Input: part model. Units: mm. Frame: model coordinates. Give positions to 0.01 mm unless a question says otherwise; leave off trailing zeros. Loops run counter-clockwise (first coordinate to the right, second up) from the corner with the lowest first, then second, coordinate; pieces in that order, holes last.
Autodesk Inventor part; units mm, degrees
ref_plane "YZ Plane" through (0, 0, 0) normal (1, 0, 0) x (0, 1, 0)
ref_plane "XZ Plane" through (0, 0, 0) normal (0, 1, 0) x (-1, 0, 0)
ref_plane "XY Plane" through (0, 0, 0) normal (0, 0, 1) x (1, 0, 0)
sketch "スケッチ1" plane through (0, 0, 0) normal (0, 0, 1) x (1, 0, 0)
  line L0 (-18.5, 36) -> (18.5, 36)
  line L1 (18.5, 36) -> (18.5, 0)
  line L2 (18.5, 0) -> (-18.5, 0)
  line L3 (-18.5, 0) -> (-18.5, 36)
  circle A0 centre (0, 4) radius 1.6
  circle A1 centre (14, 32) radius 1.6
  circle A2 centre (-14, 32) radius 1.6
  line L4 (0, 42.25) -> (0, -4.7356) construction
  point P0 (0, 0)
  point P1 (0, 0)
  dimension "d0" = 37
  dimension "d1" = 36
  dimension "d2" = 3.2
  dimension "d3" = 4
  dimension "d4" = 4
  dimension "d5" = 4.5
extrude "押し出し1" add sketch "スケッチ1" along normal blind 1.6
properties part number "PCB-EncoderMain"
(1) Ray query, probe 1 along Y at (x, z) = (14, 0.95); probe 2 along Y at (x, z) = (0, 0.9); probe 3 along X at (y, z) = (3, 0.55). Return the intervals inside material, ascending.
Values follow:
probe 1: y = 0 to 30.4, 33.6 to 36
probe 2: y = 0 to 2.4, 5.6 to 36
probe 3: x = -18.5 to -1.25, 1.25 to 18.5
(2) Cut plane B-B (x = 0). Return the cut outline in (y, z).
Values follow:
outline: (0, 0) - (2.4, 0) - (2.4, 1.6) - (0, 1.6) - close; (5.6, 0) - (36, 0) - (36, 1.6) - (5.6, 1.6) - close
(3) Pin query (flat end, axial travel): pin 1 Ø3 at (x, y) = (14, 32) entering from -Z. Return the tip coordinate at first contact, or that it passes through.
Values follow:
pin 1: passes through
(4) Cut plane A-A (y = 4). Return the cut outline in (x, z), and give its area (3 significant figures).
Values follow:
outline: (-18.5, 0) - (-1.6, 0) - (-1.6, 1.6) - (-18.5, 1.6) - close; (1.6, 0) - (18.5, 0) - (18.5, 1.6) - (1.6, 1.6) - close
area: 54.1 mm2
(5) Cut plane C-C (z = 1.15). Return the cut outline in (x, y).
Values follow:
outline: (-18.5, 0) - (18.5, 0) - (18.5, 36) - (-18.5, 36) - close; hole circle Ø3.2 at (-14, 32); hole circle Ø3.2 at (0, 4); hole circle Ø3.2 at (14, 32)
(6) Mould query, pull axis X, two halves, no side actions, for faces 1 (the flat face through (18.5, 18, 1)), 2 (the cylindrical face through (-15.6, 31.93, 0.79)), 3 (the flat face through (-18.5, 18, 1)), 4 (the flat face through (0, 0, 1)). Classes: +X half, -X half, draft (parallel to the pull), parting line (faces both ways), or undercut.
Values follow:
face 1: +X half
face 2: undercut
face 3: -X half
face 4: draft
